```python
from build123d import *

# Parameters (mm, degrees)
SKETCH1_R           = 25
BOSS_EXTRUDE1_DEPTH = 5.87
SKETCH2_R           = 16.675
CUT_EXTRUDE1_DEPTH  = 6.87
SKETCH3_R           = 21.184132597
CUT_EXTRUDE2_DEPTH  = 2


with BuildPart() as part:
    # Sketch1 → Boss-Extrude1 (new body)
    with BuildSketch(Plane.XY):
        Circle(SKETCH1_R)
    extrude(amount=BOSS_EXTRUDE1_DEPTH)

    # Sketch2 → Cut-Extrude1 (cut, through all)
    with BuildSketch(Plane(origin=(0, 0, 0), x_dir=(-1, 0, 0), z_dir=(0, 0, -1))):
        Circle(SKETCH2_R)
    extrude(amount=-CUT_EXTRUDE1_DEPTH, mode=Mode.SUBTRACT)

    # Sketch3 → Cut-Extrude2 (cut)
    with BuildSketch(Plane.XY.offset(5.87)):
        Circle(SKETCH3_R)
    extrude(amount=-CUT_EXTRUDE2_DEPTH, mode=Mode.SUBTRACT)


solid = part.part
```
Geometry check sheet. Reference: the model listing, model coordinates, mm. A direction names the side the tool comes from. Coordinates: 2 decimals unless noted, no trailing zeros. Loops run counter-clockwise (first coordinate to the right, second up) from the corner with the lowest first, then second, coordinate; pieces in that order, holes last. Notation, with made-up numbers: (-5.75, 66.5) -> (24.25, 66.5) arc R14 ccw to (24.25, 87.5) -> close; hole circle Ø9 at (82.25, 27). An arc over 180 degrees is marked (long way). Put each result on its own line as item: value.
1) Thickness scan on line 1 (Y direction, x = 0, z = 2.6) (3 decimals); line 2 (Y direction, x = 0, z = 4.8); line 3 (Z direction, x = -5.5, y = -16). Record the ranges inside material, lowest first.
Result set:
line 1: y = -25 to -16.675, 16.675 to 25
line 2: y = -25 to -21.18, 21.18 to 25
line 3: z = 0 to 3.87
2) Cross-section at A-A on x = 0. Record the boundary of the cut face in (y, z) (3 decimals).
Result set:
outline: (-25, 0) -> (-16.675, 0) -> (-16.675, 3.87) -> (-21.184, 3.87) -> (-21.184, 5.87) -> (-25, 5.87) -> close; (16.675, 0) -> (25, 0) -> (25, 5.87) -> (21.184, 5.87) -> (21.184, 3.87) -> (16.675, 3.87) -> close
3) Release check for a two-part mould opening along Y. For faces 1 (the flat face through (6, -16, 3.87)), 2 (the flat face through (-19, 11, 5.87)), 3 (the cylindrical face through (23.846, 7.509, 2.894)) record: released by +Y, released by -Y, zero draft, split by the parting line, or undercut.
Result set:
face 1: undercut
face 2: zero draft
face 3: split by the parting line
4) Cross-section at D-D on x = 19.5. Record the boundary of the cut face in (y, z).
Result set:
outline: (-15.64, 0) -> (15.64, 0) -> (15.64, 5.87) -> (8.28, 5.87) -> (8.28, 3.87) -> (-8.28, 3.87) -> (-8.28, 5.87) -> (-15.64, 5.87) -> close
5) Gauge pin test, flat ends, axial feed: pin 1 Ø1.5 at (x, y) = (-12.5, 14.5) entering from +Z; pin 2 Ø1 at (y, z) = (-4.5, 2.5) entering from +X; pin 3 Ø1.5 at (y, z) = (-19, 1) entering from +X. Record the tip position at first contact, or that the pin passes through.
Result set:
pin 1: stops at z = 3.87
pin 2: stops at x = 24.68
pin 3: stops at x = 17.09
6) Tool access check on faces 4 (the cylindrical face through (13.23, -10.15, 1.91)), 5 (the cylindrical face through (11.39, 17.86, 4.88)). Record the directions out of +Z, -Z, +X, -X, +Y, -Y that give a thin tool (end or side, any length) a straight path to the whole face; none if there is none.
Result set:
face 4: +Z, -Z
face 5: +Z
7) Cross-section at C-C on z = 1.95. Record the boundary of the cut face in (x, y) (3 decimals), plus the area to 3 significant figures.
Result set:
outline: circle Ø50 at (0, 0); hole circle Ø33.35 at (0, 0)
area: 1,090 mm^2
